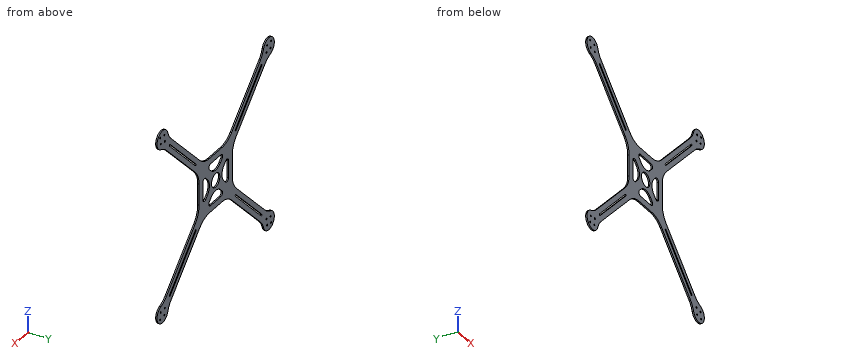
```python
from build123d import *

# Parameters (mm, degrees)
BOSS_EXTRUDE1_DEPTH     = 3.175
SKETCH4_R               = 1.905
CUT_EXTRUDE1_DEPTH      = 318.018940562
CIRPATTERN1_COUNT       = 4
CUT_EXTRUDE2_DEPTH      = 318.018940562
CUT_EXTRUDE4_DEPTH      = 318.018940562
CUT_EXTRUDE5_DEPTH      = 318.018940562
CUT_EXTRUDE5_DEPTH_BACK = 318.018940562
SKETCH9_R               = 15.875
CIRPATTERN2_COUNT       = 4


with BuildPart() as part:
    # Sketch3 → Boss-Extrude1 (new body)
    with BuildSketch(Plane(origin=(0, 0, 0), x_dir=(1, 0, 0), z_dir=(0, 1, 0))):
        with BuildLine():
            Line((-24.497438789, -63.5), (24.497438789, -63.5))
            ThreePointArc((24.497438789, -63.5), (43.937757153, -67.366919748), (60.418463274, -78.378975516))
            Line((60.418463274, -78.378975516), (170.592111486, -188.552623728))
            ThreePointArc((170.592111486, -188.552623728), (178.158900465, -198.21626677), (183.187131602, -209.412658327))
            ThreePointArc((183.187131602, -209.412658327), (218.0174226, -218.0174226), (209.412658327, -183.187131602))
            ThreePointArc((209.412658327, -183.187131602), (198.21626677, -178.158900465), (188.552623728, -170.592111486))
            Line((188.552623728, -170.592111486), (78.378975516, -60.418463274))
            ThreePointArc((78.378975516, -60.418463274), (67.366919748, -43.937757153), (63.5, -24.497438789))
            Line((63.5, -24.497438789), (63.5, 24.497438789))
            ThreePointArc((63.5, 24.497438789), (67.366919748, 43.937757153), (78.378975516, 60.418463274))
            Line((78.378975516, 60.418463274), (188.552623728, 170.592111486))
            ThreePointArc((188.552623728, 170.592111486), (198.21626677, 178.158900465), (209.412658327, 183.187131602))
            ThreePointArc((209.412658327, 183.187131602), (218.0174226, 218.0174226), (183.187131602, 209.412658327))
            ThreePointArc((183.187131602, 209.412658327), (178.158900465, 198.21626677), (170.592111486, 188.552623728))
            Line((170.592111486, 188.552623728), (60.418463274, 78.378975516))
            ThreePointArc((60.418463274, 78.378975516), (43.937757153, 67.366919748), (24.497438789, 63.5))
            Line((24.497438789, 63.5), (-24.497438789, 63.5))
            ThreePointArc((-24.497438789, 63.5), (-43.937757153, 67.366919748), (-60.418463274, 78.378975516))
            Line((-60.418463274, 78.378975516), (-170.592111486, 188.552623728))
            ThreePointArc((-170.592111486, 188.552623728), (-178.158900465, 198.21626677), (-183.187131602, 209.412658327))
            ThreePointArc((-183.187131602, 209.412658327), (-218.0174226, 218.0174226), (-209.412658327, 183.187131602))
            ThreePointArc((-209.412658327, 183.187131602), (-198.21626677, 178.158900465), (-188.552623728, 170.592111486))
            Line((-188.552623728, 170.592111486), (-78.378975516, 60.418463274))
            ThreePointArc((-78.378975516, 60.418463274), (-67.366919748, 43.937757153), (-63.5, 24.497438789))
            Line((-63.5, 24.497438789), (-63.5, -24.497438789))
            ThreePointArc((-63.5, -24.497438789), (-67.366919748, -43.937757153), (-78.378975516, -60.418463274))
            Line((-78.378975516, -60.418463274), (-188.552623728, -170.592111486))
            ThreePointArc((-188.552623728, -170.592111486), (-198.21626677, -178.158900465), (-209.412658327, -183.187131602))
            ThreePointArc((-209.412658327, -183.187131602), (-218.0174226, -218.0174226), (-183.187131602, -209.412658327))
            ThreePointArc((-183.187131602, -209.412658327), (-178.158900465, -198.21626677), (-170.592111486, -188.552623728))
            Line((-170.592111486, -188.552623728), (-60.418463274, -78.378975516))
            ThreePointArc((-60.418463274, -78.378975516), (-43.937757153, -67.366919748), (-24.497438789, -63.5))
        make_face()
    extrude(amount=BOSS_EXTRUDE1_DEPTH)

    # Sketch4 → Cut-Extrude1 (cut, through all)
    with BuildSketch(Plane(origin=(0, 3.175, 0), x_dir=(1, 0, 0), z_dir=(0, 1, 0))):
        with Locations(Location((194.399349001, 194.399349001, 0), (0, 0, 270))):
            Circle(SKETCH4_R)
        with Locations(Location((209.935192091, 196.464807909, 0), (0, 0, 270))):
            Circle(SKETCH4_R)
        with Locations(Location((212.000650999, 212.000650999, 0), (0, 0, 270))):
            Circle(SKETCH4_R)
        with Locations(Location((196.464807909, 209.935192091, 0), (0, 0, 270))):
            Circle(SKETCH4_R)
    cut_extrude1 = extrude(amount=-CUT_EXTRUDE1_DEPTH, mode=Mode.SUBTRACT)

    # CirPattern1: Cut-Extrude1 ×4 about axis
    cirpattern1_axis = Axis((0, 0, 0), (0, 1, 0))
    for i in range(1, CIRPATTERN1_COUNT):
        add(cut_extrude1.rotate(cirpattern1_axis, i * 360 / CIRPATTERN1_COUNT), mode=Mode.SUBTRACT)

    # Sketch5 → Cut-Extrude2 (cut, through all)
    with BuildSketch(Plane(origin=(0, 3.175, 0), x_dir=(1, 0, 0), z_dir=(0, 1, 0))):
        Polygon((74.212074237, 76.63674339), (175.04689706, 177.471566213), (177.471566213, 175.04689706), (76.63674339, 74.212074237), align=None)
    cut_extrude2 = extrude(amount=-CUT_EXTRUDE2_DEPTH, mode=Mode.SUBTRACT)

    # Sketch8 → Cut-Extrude4 (cut, through all)
    with BuildSketch(Plane(origin=(0, 3.175, 0), x_dir=(1, 0, 0), z_dir=(0, 1, 0))):
        with BuildLine():
            Line((-38.184603855, -24.584989879), (-31.467798631, -17.895778814))
            ThreePointArc((-31.467798631, -17.895778814), (-23.991357843, 0.049382407), (-31.393861052, 18.025169576))
            Line((-31.393861052, 18.025169576), (-38.16611946, 24.825364729))
            ThreePointArc((-38.16611946, 24.825364729), (-45.089480956, 26.213621224), (-49.015480206, 20.344488378))
            Line((-49.015480206, 20.344488378), (-49.015480206, -20.085629132))
            ThreePointArc((-49.015480206, -20.085629132), (-45.101556475, -25.949760135), (-38.184603855, -24.584989879))
        make_face()
        with BuildLine():
            Line((-20.142290993, -48.814113494), (19.88508968, -48.814113494))
            ThreePointArc((19.88508968, -48.814113494), (25.749220683, -44.900189762), (24.384450426, -37.983237143))
            Line((24.384450426, -37.983237143), (17.895778814, -31.467798631))
            ThreePointArc((17.895778814, -31.467798631), (-0.049382407, -23.991357843), (-18.025169576, -31.393861052))
            Line((-18.025169576, -31.393861052), (-24.623167344, -37.964752748))
            ThreePointArc((-24.623167344, -37.964752748), (-26.011423839, -44.888114243), (-20.142290993, -48.814113494))
        make_face()
        with BuildLine():
            Line((-19.88508968, 48.814113494), (20.142290993, 48.814113494))
            ThreePointArc((20.142290993, 48.814113494), (26.011423839, 44.888114243), (24.623167344, 37.964752748))
            Line((24.623167344, 37.964752748), (18.025169576, 31.393861052))
            ThreePointArc((18.025169576, 31.393861052), (0.049382407, 23.991357843), (-17.895778814, 31.467798631))
            Line((-17.895778814, 31.467798631), (-24.384450426, 37.983237143))
            ThreePointArc((-24.384450426, 37.983237143), (-25.749220683, 44.900189762), (-19.88508968, 48.814113494))
        make_face()
        with BuildLine():
            Line((49.015480206, -20.344488378), (49.015480206, 20.085629132))
            ThreePointArc((49.015480206, 20.085629132), (45.101556475, 25.949760135), (38.184603855, 24.584989879))
            Line((38.184603855, 24.584989879), (31.467798631, 17.895778814))
            ThreePointArc((31.467798631, 17.895778814), (23.991357843, -0.049382407), (31.393861052, -18.025169576))
            Line((31.393861052, -18.025169576), (38.16611946, -24.825364729))
            ThreePointArc((38.16611946, -24.825364729), (45.089480956, -26.213621224), (49.015480206, -20.344488378))
        make_face()
    extrude(amount=-CUT_EXTRUDE4_DEPTH, mode=Mode.SUBTRACT)

    # Sketch9 → Cut-Extrude5 (cut, two sides: drawn at the far end of the back side and taken through both)
    with BuildSketch(Plane(origin=(0, 3.175, 0), x_dir=(1, 0, 0), z_dir=(0, 1, 0)).offset(-CUT_EXTRUDE5_DEPTH_BACK)):
        with Locations(Location((0, 0, 0), (0, 0, 270))):
            Circle(SKETCH9_R)
    extrude(amount=CUT_EXTRUDE5_DEPTH + CUT_EXTRUDE5_DEPTH_BACK, mode=Mode.SUBTRACT)

    # CirPattern2: Cut-Extrude2 ×4 about axis
    cirpattern2_axis = Axis((0, 0, 0), (0, 1, 0))
    for i in range(1, CIRPATTERN2_COUNT):
        add(cut_extrude2.rotate(cirpattern2_axis, i * 360 / CIRPATTERN2_COUNT), mode=Mode.SUBTRACT)


solid = part.part
```
The model under review builds one solid part; all positions refer to its coordinate system, in mm. Round coordinates to 2 decimals unless told otherwise and drop trailing zeros. Write each loop counter-clockwise with the first axis right and the second up, starting at its lowest first coordinate (ties: lowest second). Pieces come first, ordered by that corner, then holes.
(1) We need section A-A on z = 0. Give the boundary of the cut face in (x, y) (1 decimal), and give its area (3 significant figures).
(2) Wall thickness on L1, parallel to X at y = 0.9, z = -170.5; L2, parallel to X at y = 1.35, z = 19; L3, parallel to X at y = 2.2, z = 105.5: over which ranges is each line inside the solid? List them lowest first.
(3) We need section C-C on y = 1.2. Give the number of separate pieces and of enclosed holes in the cut face, and give its area (3 significant figures).
(4) We need section B-B on x = 0. Give the boundary of the cut face in (y, z) (1 decimal).
(5) Insertion check: pin 1 (1 mm diameter, centred on x = -30, y = 2, fed in from +Z); pin 2 (3 mm diameter, centred on x = 194.4, z = 194.4, fed in from +Y); pin 3 (1.6 mm diameter, centred on y = 1.5, z = -8.5, fed in from +X). Each pin has a flat end and moves straight along its axis. Give the tip position at first contact, or say it passes through.
Findings below:
1. outline: (-63.5, 0) - (-49, 0) - (-49, 3.2) - (-63.5, 3.2) - close; (-24, 0) - (-15.9, 0) - (-15.9, 3.2) - (-24, 3.2) - close; (15.9, 0) - (24, 0) - (24, 3.2) - (15.9, 3.2) - close; (49, 0) - (63.5, 0) - (63.5, 3.2) - (49, 3.2) - close
1. area: 144 mm2
2. L1: x = -188.46 to -172.92, -168.08 to -152.54, 152.54 to 168.08, 172.92 to 188.46
2. L2: x = -63.5 to -49.02, -32.58 to 32.36, 49.02 to 63.5
2. L3: x = -123.46 to -107.92, -103.08 to -87.54, 87.54 to 103.08, 107.92 to 123.46
3. separate pieces: 1
3. enclosed holes: 25
3. area: 34,000 mm2
4. outline: (0, -63.5) - (3.2, -63.5) - (3.2, -48.8) - (0, -48.8) - close; (0, -24) - (3.2, -24) - (3.2, -15.9) - (0, -15.9) - close; (0, 15.9) - (3.2, 15.9) - (3.2, 24) - (0, 24) - close; (0, 48.8) - (3.2, 48.8) - (3.2, 63.5) - (0, 63.5) - close
5. pin 1: stops at z = 63.86
5. pin 2: passes through
5. pin 3: stops at x = 63.5
